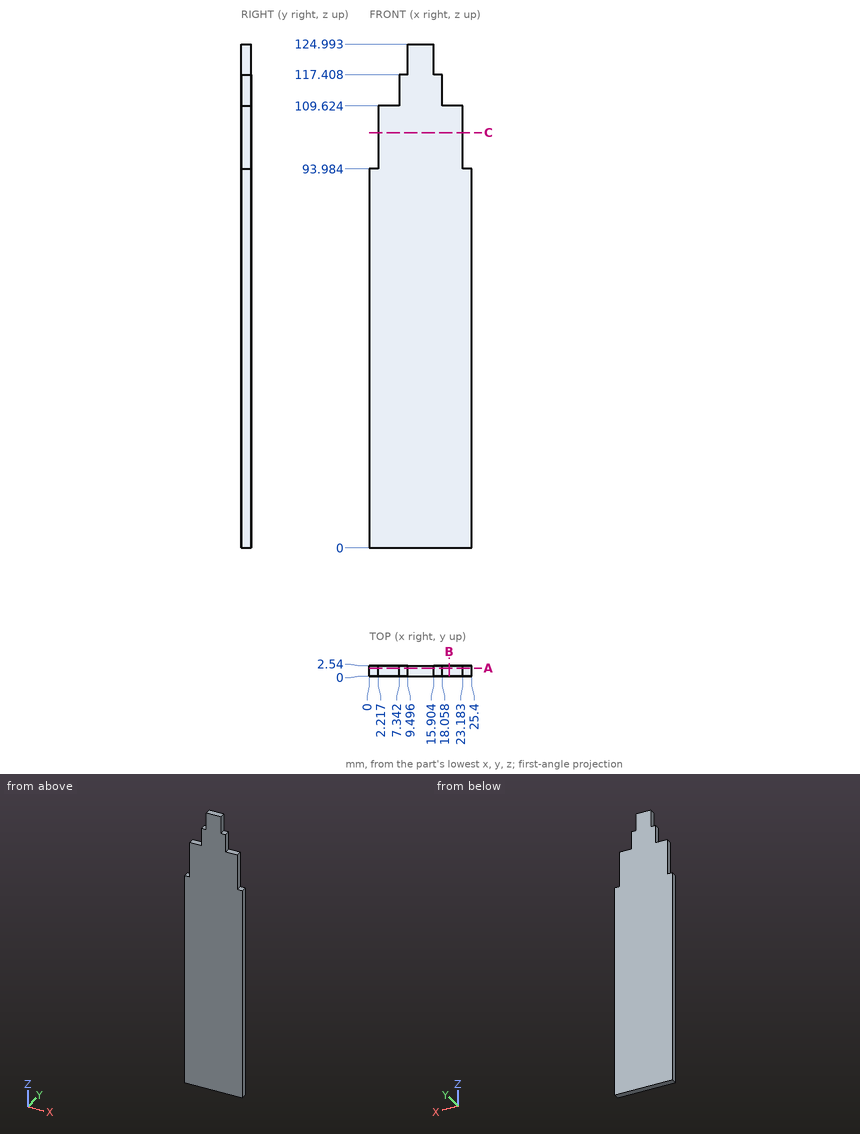
Check sheet for the drawn part. Datum: minimum x, y, z corner. Units: mm. Round coordinates to 2 decimals unless told otherwise and drop trailing zeros. Write each loop counter-clockwise with the first axis right and the second up, starting at its lowest first coordinate (ties: lowest second). Pieces come first, ordered by that corner, then holes. Notation, with made-up numbers: (-12.5, 28.25) -> (44.5, 28.25) arc R6 ccw to (44.5, 33.25) -> close; hole circle Ø1 at (-10, 50). An arc over 180 degrees is marked (long way). Write each question's results on one line, items separated by ' | '. Start each with the question number.
1. Cross-section at A-A (y = 1.95). Enter the section's corners in (x, z) (1 decimal), then the cut area to 3 significant figures.
2. Cross-section at C-C (z = 103). Enter the section's corners in (x, y).
3. Cross-section at B-B (x = 19.75). Enter the section's corners in (y, z) (1 decimal).
4. Material ranges on probe 1 along Z at (x, y) = (2, 0.25); probe 2 along Z at (x, y) = (4.75, 1.5) (1 decimal); probe 3 along X at (y, z) = (2.45, 110), recorded low to high. Write a range as from..to.
5. Depth check by flat-ended pin: P1, Ø1.3, axis at y = 1.5, z = 112.5, coming from the -X side; P2, Ø1.3, axis at x = 19.5, y = 1.5, coming from the +Z side; P3, Ø0.8, axis at y = 1, z = 123, coming from the -X side (1 decimal). Enter the tip coordinate at first touch or a pass-through.
Solutions:
1) outline: (0, 0) -> (25.4, 0) -> (25.4, 94) -> (23.2, 94) -> (23.2, 109.6) -> (18.1, 109.6) -> (18.1, 117.4) -> (15.9, 117.4) -> (15.9, 125) -> (9.5, 125) -> (9.5, 117.4) -> (7.3, 117.4) -> (7.3, 109.6) -> (2.2, 109.6) -> (2.2, 94) -> (0, 94) -> close | area: 2,850 mm2
2) outline: (2.22, 0) -> (23.18, 0) -> (23.18, 2.54) -> (2.22, 2.54) -> close
3) outline: (0, 0) -> (2.5, 0) -> (2.5, 109.6) -> (0, 109.6) -> close
4) probe 1: z = 0..93.98 | probe 2: z = 0..109.6 | probe 3: x = 7.34..18.06
5) P1: stops at x = 7.34 | P2: stops at z = 109.62 | P3: stops at x = 9.5
